Check sheet for the modelled part. Datum: model origin and axes. Units: mm. Face numbers are marked on the shaded views. Give positions to 0.01 mm unless a question says otherwise; leave off trailing zeros. Order: outer loops, then holes, each group sorted by start corner. A loop starts at its lowest first (then second) coordinate and runs counter-clockwise, first axis right, second up.
```python
from build123d import *

# Parameters (mm, degrees)
F0_R     = 4.05
F1_DEPTH = 20


with BuildPart() as f1:
    # F0 (on Front) → F1 (new body)
    with BuildSketch(Plane.XZ):
        with BuildLine():
            Line((3.3250001364, 5.7590688564), (0, 7.6787585802))
            Line((0, 7.6787585802), (-3.3249999524, 5.7590689627))
            ThreePointArc((-3.3249999524, 5.7590689627), (1.062e-07, 6.65), (3.3250001364, 5.7590688564))
        make_face()
        with BuildLine():
            Line((6.65, 3.8393792901), (3.3250001364, 5.7590688564))
            ThreePointArc((3.3250001364, 5.7590688564), (5.7590689745, 3.3249999318), (6.65, 0))
            Line((6.65, 0), (6.65, 3.8393792901))
        make_face()
        with BuildLine():
            ThreePointArc((6.65, 0), (5.7590689745, 3.3249999318), (3.3250001364, 5.7590688564))
            ThreePointArc((3.3250001364, 5.7590688564), (1.062e-07, 6.65), (-3.3249999524, 5.7590689627))
            ThreePointArc((-3.3249999524, 5.7590689627), (-5.7590689214, 3.3250000238), (-6.65, 0))
            ThreePointArc((-6.65, 0), (-5.7590689227, -3.3250000216), (-3.3249999568, -5.7590689601))
            ThreePointArc((-3.3249999568, -5.7590689601), (2.14e-08, -6.65), (3.3249999939, -5.7590689387))
            ThreePointArc((3.3249999939, -5.7590689387), (5.7590689334, -3.3250000031), (6.65, 0))
        make_face()
        Circle(F0_R, mode=Mode.SUBTRACT)
        with BuildLine():
            ThreePointArc((-6.65, 0), (-5.7590689214, 3.3250000238), (-3.3249999524, 5.7590689627))
            Line((-3.3249999524, 5.7590689627), (-6.65, 3.8393792901))
            Line((-6.65, 3.8393792901), (-6.65, 0))
        make_face()
        with BuildLine():
            Line((6.65, -3.8393792901), (6.65, 0))
            ThreePointArc((6.65, 0), (5.7590689334, -3.3250000031), (3.3249999939, -5.7590689387))
            Line((3.3249999939, -5.7590689387), (6.65, -3.8393792901))
        make_face()
        with BuildLine():
            ThreePointArc((-3.3249999568, -5.7590689601), (-5.7590689227, -3.3250000216), (-6.65, 0))
            Line((-6.65, 0), (-6.65, -3.8393792901))
            Line((-6.65, -3.8393792901), (-3.3249999568, -5.7590689601))
        make_face()
        with BuildLine():
            Line((0, -7.6787585802), (3.3249999939, -5.7590689387))
            ThreePointArc((3.3249999939, -5.7590689387), (2.14e-08, -6.65), (-3.3249999568, -5.7590689601))
            Line((-3.3249999568, -5.7590689601), (0, -7.6787585802))
        make_face()
    extrude(amount=F1_DEPTH)


solid = f1.part
```
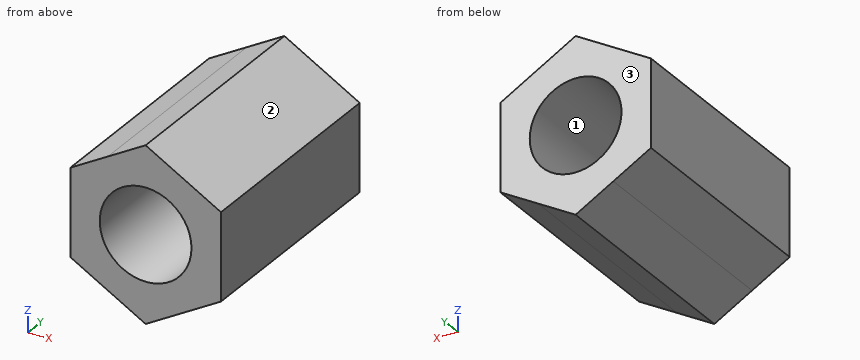
(1) Cross-section at D-D on z = 4.75. Enter the section's corners in (x, y), then the cut area to 3 significant figures.
Response values:
outline: (-5.07, -20) - (5.07, -20) - (5.07, 0) - (-5.07, 0) - close
area: 203 mm2
(2) Cross-section at B-B on y = -15.5. Enter the section's corners in (x, z) (3 decimals).
Response values:
outline: (-6.65, -3.839) - (0, -7.679) - (6.65, -3.839) - (6.65, 3.839) - (0, 7.679) - (-6.65, 3.839) - close; hole circle Ø8.1 at (0, 0)
(3) Cross-section at C-C on x = -2. Enter the section's corners in (y, z).
Response values:
outline: (-20, -6.52) - (0, -6.52) - (0, -3.52) - (-20, -3.52) - close; (-20, 3.52) - (0, 3.52) - (0, 6.52) - (-20, 6.52) - close
(4) Release check for a two-part mould opening along Z. For the marked faces 1, 2 and 3 record: released by +Z, released by -Z, zero draft, split by the parting line, or undercut.
Response values:
face 1: undercut
face 2: released by +Z
face 3: zero draft
(5) Gauge pin test, flat ends, axial feed: pin 1 Ø3 at (x, y) = (-5, -3.5) entering from +Z; pin 2 Ø4 at (x, y) = (5, -9.5) entering from -Z. Record the tip position at first contact, or that the pin passes through.
Response values:
pin 1: stops at z = 5.66
pin 2: stops at z = -5.95
(6) Cross-section at A-A on z = 0. Enter the section's corners in (x, y).
Response values:
outline: (-6.65, -20) - (-4.05, -20) - (-4.05, 0) - (-6.65, 0) - close; (4.05, -20) - (6.65, -20) - (6.65, 0) - (4.05, 0) - close
(7) Material ranges on L1, parallel to Z at x = -1.5, y = -9.5; L2, parallel to X at y = -7.5, z = 2.5; L3, parallel to Z at x = -3.5, y = -1.75, recorded low to high.
Response values:
L1: z = -6.81 to -3.76, 3.76 to 6.81
L2: x = -6.65 to -3.19, 3.19 to 6.65
L3: z = -5.66 to -2.04, 2.04 to 5.66
